Input: part model. Units: mm. Frame: model coordinates. Coordinates: 2 decimals unless noted, no trailing zeros. Order: outer loops, then holes, each group sorted by start corner. A loop starts at its lowest first (then second) coordinate and runs counter-clockwise, first axis right, second up. Notation, with made-up numbers: M 56.25,-36 L 104.25,-36 A36 ccw 104.25,-1 Z; hole C 35,-3 d7. An arc over 180 degrees is marked long. Answer in a Markdown table with one row per item.
from build123d import *

# Parameters (mm, degrees)
CROQUIS2_W              = 63.5
CROQUIS2_H              = 450
SALIENTE_EXTRUIR1_DEPTH = 63.5
CROQUIS3_R              = 19.05
SALIENTE_EXTRUIR2_DEPTH = 14
SALIENTE_EXTRUIR3_START = 14
CROQUIS4_R              = 19.05
SALIENTE_EXTRUIR3_DEPTH = 14
CROQUIS5_W              = 63.5
CROQUIS5_H              = 63.5
CROQUIS5_R              = 31
CORTAR_EXTRUIR1_DEPTH   = 12.7


with BuildPart() as part:
    # Croquis2 → Saliente-Extruir1 (new body)
    with BuildSketch(Plane.XY):
        Rectangle(CROQUIS2_W, CROQUIS2_H)
    extrude(amount=SALIENTE_EXTRUIR1_DEPTH)

    # Croquis3 → Saliente-Extruir2 (add)
    with BuildSketch(Plane.XY.offset(63.5)):
        with Locations(Location((0, -195, 0), (0, 0, 180))):
            Circle(CROQUIS3_R)
    extrude(amount=SALIENTE_EXTRUIR2_DEPTH)

    # Croquis4 → Saliente-Extruir3 (add)
    with BuildSketch(Plane(origin=(0, 0, 0), x_dir=(-1, 0, 0), z_dir=(0, 0, -1)).offset(SALIENTE_EXTRUIR3_START)):
        with Locations((0, -195)):
            Circle(CROQUIS4_R)
    extrude(amount=-SALIENTE_EXTRUIR3_DEPTH)

    # Croquis5 → Cortar-Extruir1 (cut)
    with BuildSketch(Plane(origin=(0, 225, 0), x_dir=(1, 0, 0), z_dir=(0, 1, 0))):
        with Locations((0, -31.75)):
            Rectangle(CROQUIS5_W, CROQUIS5_H)
        with Locations(Location((0, -31.75, 0), (0, 0, 270))):
            Circle(CROQUIS5_R, mode=Mode.SUBTRACT)
    extrude(amount=-CORTAR_EXTRUIR1_DEPTH, mode=Mode.SUBTRACT)


solid = part.part
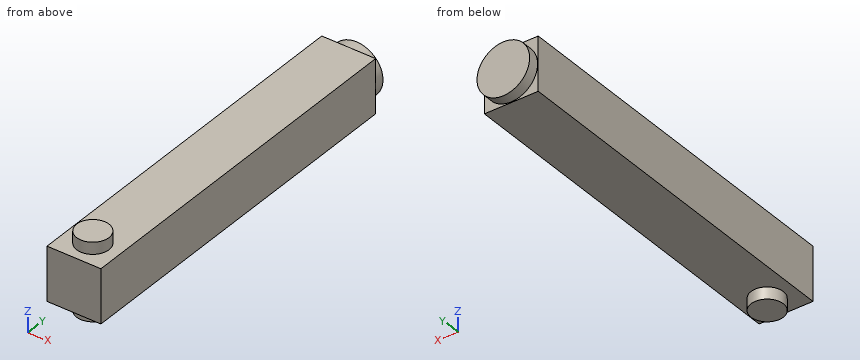
1) Material intervals for probe 1 along Z at (x, y) = (13.5, -53.5); probe 2 along Y at (x, z) = (28, 3), sorted ascending.
Resolved:
| item | result |
|---|---|
| probe 1 | z = 0 to 63.5 |
| probe 2 | y = -225 to 212.3 |
2) Cut plane A-A, the plane x = 0. Output: boundary loops of the cut face in (y, z).
Resolved:
| item | result |
|---|---|
| outline | M -225,0 L -214.05,0 L -214.05,-14 L -175.95,-14 L -175.95,0 L 212.3,0 L 212.3,0.75 L 225,0.75 L 225,62.75 L 212.3,62.75 L 212.3,63.5 L -175.95,63.5 L -175.95,77.5 L -214.05,77.5 L -214.05,63.5 L -225,63.5 Z |
3) Cut plane B-B, the plane y = -195. Output: boundary loops of the cut face in (x, z).
Resolved:
| item | result |
|---|---|
| outline | M -31.75,0 L -19.05,0 L -19.05,-14 L 19.05,-14 L 19.05,0 L 31.75,0 L 31.75,63.5 L 19.05,63.5 L 19.05,77.5 L -19.05,77.5 L -19.05,63.5 L -31.75,63.5 Z |
4) Contact query for flat-ended pins moving along their axis: pin 1 (10 mm diameter, centred on x = -3.5, y = 27.5, fed in from +Z); pin 2 (5 mm diameter, centred on x = 15, y = 83.5, fed in from -Z). Output: stop coordinate, or through.
Resolved:
| item | result |
|---|---|
| pin 1 | stops at z = 63.5 |
| pin 2 | stops at z = 0 |
5) Cut plane C-C, the plane z = -5.5. Output: boundary loops of the cut face in (x, y), and give its area (3 significant figures).
Resolved:
| item | result |
|---|---|
| outline | C 0,-195 d38.1 |
| area | 1,140 mm2 |
